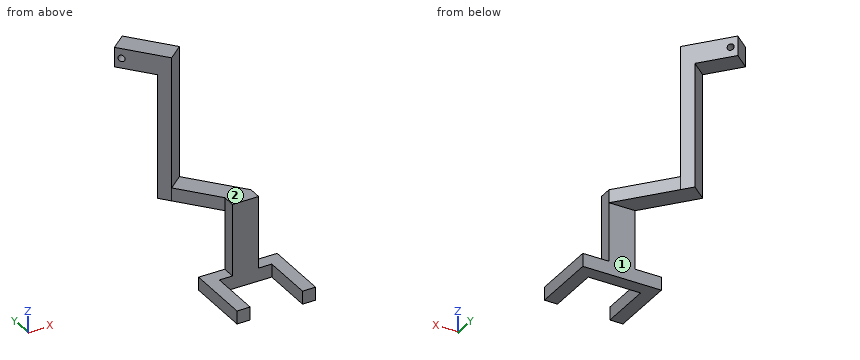
from build123d import *

# Parameters (mm, degrees)
P_IDAT_VYSUNUT_M1_DEPTH  = 10
SKICA2_W                 = 20
SKICA2_H                 = 10
P_IDAT_VYSUNUT_M2_DEPTH  = 55
P_IDAT_VYSUNUT_M3_DEPTH  = 10
SKICA4_W                 = 15.320888863
SKICA4_H                 = 110
P_IDAT_VYSUNUT_M4_DEPTH  = 10
SKICA5_W                 = 15.320888863
SKICA5_H                 = 15
P_IDAT_VYSUNUT_M5_DEPTH  = 30
SKICA6_R                 = 2.5
ODEBRAT_VYSUNUT_M1_DEPTH = 187.809937293


with BuildPart() as part:
    # Skica1 → Přidat vysunutím1 (new body)
    with BuildSketch(Plane.XY):
        Polygon((0, 0), (60, 0), (60, -50), (50, -50), (50, -10), (10, -10), (10, -50), (0, -50), align=None)
    extrude(amount=P_IDAT_VYSUNUT_M1_DEPTH)

    # Skica2 → Přidat vysunutím2 (add)
    with BuildSketch(Plane.XY.offset(10)):
        with Locations((30, -5)):
            Rectangle(SKICA2_W, SKICA2_H)
    extrude(amount=P_IDAT_VYSUNUT_M2_DEPTH)

    # Skica3 → Přidat vysunutím3 (add)
    with BuildSketch(Plane.XY.offset(65)):
        Polygon((40, 0), (7.860619516, 38.302222156), (-3.875862261, 28.454144626), (20, 0), align=None)
    extrude(amount=-P_IDAT_VYSUNUT_M3_DEPTH)

    # Skica4 → Přidat vysunutím4 (add)
    with BuildSketch(Plane(origin=(-15.612344038, 18.606067096, 0), x_dir=(0.7660444431189743, 0.6427876096865438, 0), z_dir=(-0.6427876096865438, 0.7660444431189745, 0))):
        with Locations((22.981333294, -110)):
            Rectangle(SKICA4_W, SKICA4_H)
    extrude(amount=P_IDAT_VYSUNUT_M4_DEPTH)

    # Skica5 → Přidat vysunutím5 (add)
    with BuildSketch(Plane(origin=(-22.040220135, 26.266511527, 0), x_dir=(0.7660444431189743, 0.6427876096865438, 0), z_dir=(-0.6427876096865438, 0.7660444431189745, 0))):
        with Locations((22.981333294, -157.5)):
            Rectangle(SKICA5_W, SKICA5_H)
    extrude(amount=P_IDAT_VYSUNUT_M5_DEPTH)

    # Skica6 → Odebrat vysunutím1 (cut, through all)
    with BuildSketch(Plane(origin=(23.472963553, 19.69615506, 0), x_dir=(0, 0, -1), z_dir=(0.7660444431189746, 0.6427876096865435, 0))):
        with Locations(Location((-157.5, 59.288495613, 0), (0, 0, 90))):
            Circle(SKICA6_R)
    extrude(amount=-ODEBRAT_VYSUNUT_M1_DEPTH, mode=Mode.SUBTRACT)


solid = part.part
Could you check a few things on this model? Use its own coordinates, in mm. Face numbers are marked on the shaded views. Coordinates: 2 decimals unless noted, no trailing zeros. Order: outer loops, then holes, each group sorted by start corner. A loop starts at its lowest first (then second) coordinate and runs counter-clockwise, first axis right, second up.
Q1. Suppose I cut it at D-D on x = 29. Please give me the cut outline in (y, z), and give its area (3 significant figures).
Q2. Will these pins go through, and if not, where does the flat tip stop? pin 1 (10 mm diameter, centred on x = 10, y = -36, fed in from +Z); pin 2 (8 mm diameter, centred on y = -3.5, z = 50, fed in from +X); pin 3 (4 mm diameter, centred on x = -6, y = 35, fed in from -Z).
Q3. Please list where these lines run through material, in increasing order: L1, parallel to Y at x = 30, z = 50; L2, parallel to Z at x = -9.5, y = 35.5; L3, parallel to Z at x = 28, y = 14.
Q4. Suppose I cut it at C-C on x = 12. Please give me the cut outline in (y, z), and give its area (3 significant figures).
Q5. Suppose I cut it at B-B on z = 57. Please give me the cut outline in (x, y), and give its area (3 significant figures).
Q6. Thinking about a two-plate mould opening in Z: for the marked faces 1 and 2, which applies, released by +Z, released by -Z, zero draft, split by the parting line, or undercut?
Q7. Suppose I cut it at A-A on y = -27.5. Please give me the cut outline in (x, z).
Answer:
1. outline: (-10, 0) - (0, 0) - (0, 55) - (13.11, 55) - (13.11, 65) - (-10, 65) - close
1. area: 781 mm2
2. pin 1: stops at z = 10
2. pin 2: stops at x = 40
2. pin 3: stops at z = 55
3. L1: y = -10 to 0
3. L2: z = 55 to 165
3. L3: z = 55 to 65
4. outline: (-10, 0) - (0, 0) - (0, 10) - (-10, 10) - close; (9.53, 55) - (33.37, 55) - (33.37, 65) - (9.53, 65) - close
4. area: 338 mm2
5. outline: (-10.3, 36.11) - (20, 0) - (20, -10) - (40, -10) - (40, 0) - (1.43, 45.96) - close
5. area: 1,020 mm2
6. face 1: zero draft
6. face 2: released by +Z
7. outline: (0, 0) - (10, 0) - (10, 10) - (0, 10) - close; (50, 0) - (60, 0) - (60, 10) - (50, 10) - close
